Answer from the drawing. Dimensions are ordinates in mm from the lowest x, y and z of the part. A direction names the side the tool comes from. Coordinates: 2 decimals unless noted, no trailing zeros. Write each loop counter-clockwise with the first axis right and the second up, starting at its lowest first coordinate (ties: lowest second). Pieces come first, ordered by that corner, then holes.
(1) Section A-A on y = 8 is taken. Write down the section's boundary in (x, z), then the cut area to 3 significant figures.
(2) Given pin 1 (8 mm diameter, centred on y = 13.5, z = 12, fed in from -X); pin 2 (12 mm diameter, centred on x = 24.5, z = 19.5, fed in from +Y); pin 3 (0.8 mm diameter, centred on x = 32, z = 11, fed in from +Y); pin 4 (12 mm diameter, centred on x = 11.5, y = 13.5, fed in from +Z), each flat-ended and moving along its own axis, determine where each tip first touches the part or whether it passes through.
(3) Section B-B on z = 12 is taken. State how many separate pieces and enclosed holes the cut face has.
(4) Section D-D on y = 17.25 is taken. Write down the section's boundary in (x, z), then the cut area to 3 significant figures.
(5) Find the intervals of material crossed by probe 1 along X at (y, z) = (11.75, 2.75); probe 2 along Y at (x, z) = (32.1, 12) (1 decimal); probe 3 along Z at (x, y) = (32.25, 13.5) (3 decimals), in increasing order.
(6) Section C-C on y = 13.5 is taken. Write down the section's boundary in (x, z) (3 decimals).
(7) The mould has two halves that part along X. Classify the marked faces 3, 4, 5 and 6: +X half, -X half, draft (parallel to the pull), parting line (faces both ways), or undercut.
(8) Which of the six approach directions +Z, -Z, +X, -X, +Y, -Y give full straight-line access (tool end or side, diameter ignored) to the marked faces 1 and 2?
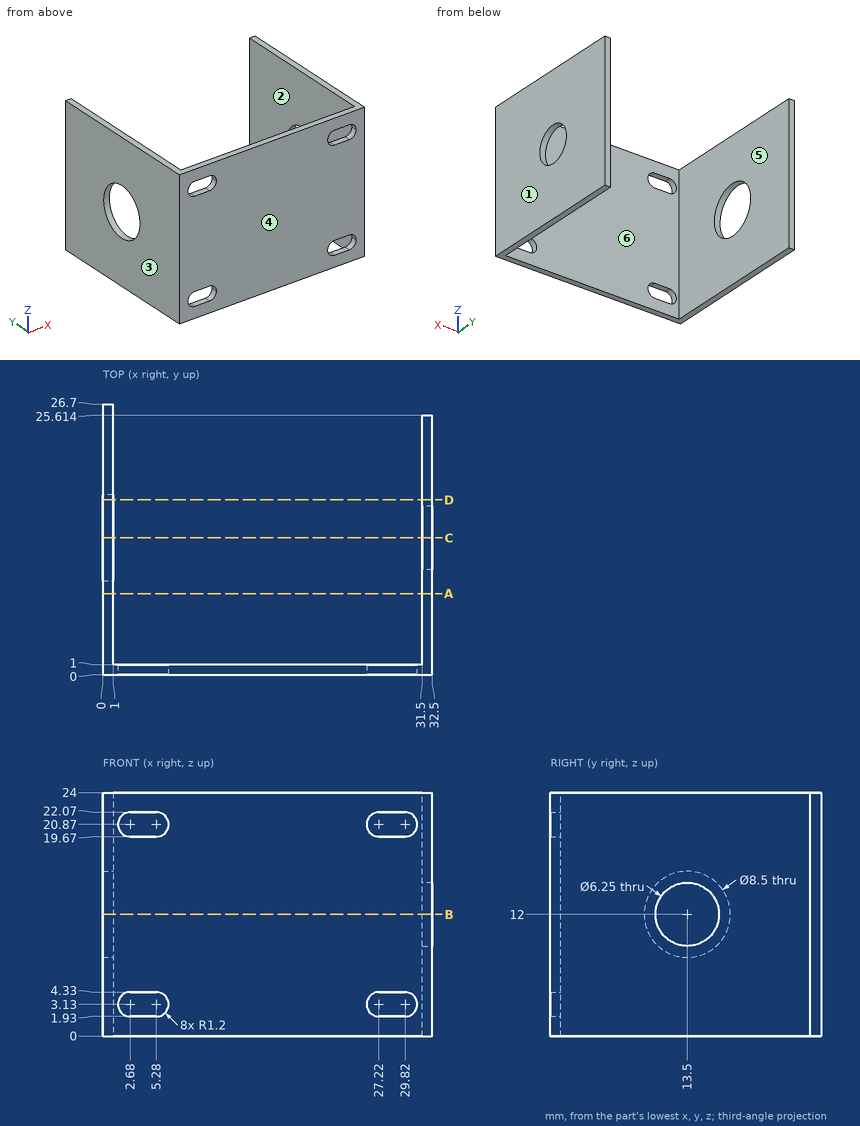
Response:
1. outline: (0, 0) - (1, 0) - (1, 24) - (0, 24) - close; (31.5, 0) - (32.5, 0) - (32.5, 24) - (31.5, 24) - close
1. area: 48.0 mm2
2. pin 1: stops at x = 31.5
2. pin 2: stops at y = 1
2. pin 3: stops at y = 25.61
2. pin 4: passes through
3. separate pieces: 3
3. enclosed holes: 0
4. outline: (0, 0) - (1, 0) - (1, 10) - (0, 10) - close; (0, 14) - (1, 14) - (1, 24) - (0, 24) - close; (31.5, 0) - (32.5, 0) - (32.5, 24) - (31.5, 24) - close
4. area: 44.0 mm2
5. probe 1: x = 0 to 1, 31.5 to 32.5
5. probe 2: y = 0 to 10.4, 16.6 to 25.6
5. probe 3: z = 0 to 8.875, 15.125 to 24
6. outline: (0, 0) - (1, 0) - (1, 7.75) - (0, 7.75) - close; (0, 16.25) - (1, 16.25) - (1, 24) - (0, 24) - close; (31.5, 0) - (32.5, 0) - (32.5, 8.875) - (31.5, 8.875) - close; (31.5, 15.125) - (32.5, 15.125) - (32.5, 24) - (31.5, 24) - close
7. face 3: -X half
7. face 4: draft
7. face 5: undercut
7. face 6: undercut
8. face 1: +Z, -Z, +X, +Y, -Y
8. face 2: +Z, -Z, +Y
